from build123d import *

# Parameters (mm, degrees)
SKETCH1_R           = 53.18125
BOSS_EXTRUDE1_DEPTH = 50.8
SKETCH2_R           = 50.8
SKETCH2_R_2         = 47.625
BOSS_EXTRUDE2_DEPTH = 12.7
SKETCH3_R           = 50.00625
CUT_EXTRUDE1_DEPTH  = 53.34
CUT_EXTRUDE1_DRAFT  = -5
SKETCH4_R           = 3.302
CUT_EXTRUDE2_DEPTH  = 93.204372473
SKETCH5_R           = 1.7859375
CUT_EXTRUDE3_DEPTH  = 10.16
CIRPATTERN1_COUNT   = 8


with BuildPart() as part:
    # Sketch1 → Boss-Extrude1 (new body)
    with BuildSketch(Plane(origin=(0, 0, 0), x_dir=(1, 0, 0), z_dir=(0, 1, 0))):
        with Locations(Location((0, 0, 0), (0, 0, 270))):
            Circle(SKETCH1_R)
    extrude(amount=BOSS_EXTRUDE1_DEPTH)

    # Sketch2 → Boss-Extrude2 (add)
    with BuildSketch(Plane.XZ):
        with Locations(Location((0, 0, 0), (0, 0, 270))):
            Circle(SKETCH2_R)
        Circle(SKETCH2_R_2, mode=Mode.SUBTRACT)
        Circle(SKETCH2_R_2)
    extrude(amount=BOSS_EXTRUDE2_DEPTH)


with BuildPart() as cut_extrude1_tool:
    # Sketch3 → Cut-Extrude1 (with draft: the straight prism first)
    with BuildSketch(Plane(origin=(0, 50.8, 0), x_dir=(1, 0, 0), z_dir=(0, 1, 0))):
        Circle(SKETCH3_R)
    extrude(amount=-CUT_EXTRUDE1_DEPTH)
    # Cut-Extrude1: the draft: its side faces are tilted about the plane it starts from
    cut_extrude1_sides = [cut_extrude1_tool.faces().sort_by_distance(p)[0] for p in [
        (-50.00625, 24.13, 0),
    ]]
    draft(cut_extrude1_sides, Plane(origin=(0, 50.8, 0), x_dir=(1, 0, 0), z_dir=(0, 1, 0)), CUT_EXTRUDE1_DRAFT)


with BuildPart() as part_1:
    add(part.part)

    # Cut-Extrude1: cut by cut_extrude1_tool
    add(cut_extrude1_tool.part, mode=Mode.SUBTRACT)

    # Sketch4 → Cut-Extrude2 (cut, through all)
    with BuildSketch(Plane(origin=(0, -2.54, 0), x_dir=(1, 0, 0), z_dir=(0, 1, 0))):
        with Locations(Location((0, 0, 0), (0, 0, 270))):
            Circle(SKETCH4_R)
    extrude(amount=-CUT_EXTRUDE2_DEPTH, mode=Mode.SUBTRACT)

    # Sketch5 → Cut-Extrude3 (cut)
    with BuildSketch(Plane(origin=(50.8, 0, 0), x_dir=(0, 0, -1), z_dir=(1, 0, 0))):
        with Locations((0, -5.35305)):
            Circle(SKETCH5_R)
    cut_extrude3 = extrude(amount=-CUT_EXTRUDE3_DEPTH, mode=Mode.SUBTRACT)

    # CirPattern1: Cut-Extrude3 ×8 about axis
    cirpattern1_axis = Axis((0, 0, 0), (0, 1, 0))
    for i in range(1, CIRPATTERN1_COUNT):
        add(cut_extrude3.rotate(cirpattern1_axis, i * 360 / CIRPATTERN1_COUNT), mode=Mode.SUBTRACT)


solid = part_1.part
For this review, take the finished solid that the model builds, in its own axes (mm). A direction names the side the tool comes from. Give positions to 0.01 mm unless a question says otherwise; leave off trailing zeros. Loops run counter-clockwise (first coordinate to the right, second up) from the corner with the lowest first, then second, coordinate; pieces in that order, holes last. Notation, with made-up numbers: (74, 50.25) -> (114, 50.25) arc R22 ccw to (114, 74.25) -> close; hole circle Ø1 at (78, 88). An arc over 180 degrees is marked (long way). One line per question, with ' | ' between items.
1) We need section A-A (z = 0). Write out the cut boundary in (x, y), plus the area to 3 significant figures.
Resolved:
outline: (-53.18, 0) -> (-50.8, 0) -> (-50.8, -3.57) -> (-40.64, -3.57) -> (-40.64, -7.14) -> (-50.8, -7.14) -> (-50.8, -12.7) -> (-3.3, -12.7) -> (-3.3, -2.54) -> (-45.34, -2.54) -> (-50.01, 50.8) -> (-53.18, 50.8) -> close; (3.3, -12.7) -> (50.8, -12.7) -> (50.8, -7.14) -> (40.64, -7.14) -> (40.64, -3.57) -> (50.8, -3.57) -> (50.8, 0) -> (53.18, 0) -> (53.18, 50.8) -> (50.01, 50.8) -> (45.34, -2.54) -> (3.3, -2.54) -> close | area: 1,470 mm2
2) We need section B-B (x = 0). Write out the cut boundary in (y, z), plus the area to 3 significant figures.
Resolved:
outline: (-12.7, -50.8) -> (-7.14, -50.8) -> (-7.14, -40.64) -> (-3.57, -40.64) -> (-3.57, -50.8) -> (0, -50.8) -> (0, -53.18) -> (50.8, -53.18) -> (50.8, -50.01) -> (-2.54, -45.34) -> (-2.54, -3.3) -> (-12.7, -3.3) -> close; (-12.7, 3.3) -> (-2.54, 3.3) -> (-2.54, 45.34) -> (50.8, 50.01) -> (50.8, 53.18) -> (0, 53.18) -> (0, 50.8) -> (-3.57, 50.8) -> (-3.57, 40.64) -> (-7.14, 40.64) -> (-7.14, 50.8) -> (-12.7, 50.8) -> close | area: 1,470 mm2
3) For faces 4 (the flat face through (0, -5, 40.64)), 5 (the flat face through (40.64, -5, 0)), 6 (the cylindrical face through (-45.79, -6.94, 0.82)), list the 3-axis set-ups (+Z, -Z, +X, -X, +Y, -Y) from which the entire face can be reached by the end or side of a thin tool; tool diameter is ignored.
Resolved:
face 4: +Z | face 5: +X | face 6: -X
4) We need section C-C (y = 11). Write out the cut boundary in (x, z), plus the area to 3 significant figures.
Resolved:
outline: circle Ø106.36 at (0, 0); hole circle Ø93.05 at (0, 0) | area: 2,090 mm2
5) The part is to be moulded in two halves that separate along Z. For faces 1 (the conical face through (-10.229, 18.577, 46.065)), 2 (the flat face through (1, -12.7, -11)), 3 (the flat face through (0, -5, -40.64)), say which applies: +Z half, -Z half, draft (parallel to the pull), parting line (faces both ways), or undercut.
Resolved:
face 1: undercut | face 2: draft | face 3: -Z half
6) To check wall thickness, follow probe 1 along Y at (x, z) = (35.5, 37.5); probe 2 along X at (y, z) = (4, 32); probe 3 along X at (y, z) = (-6, 42). State the ranges of each line that lie inside material, in increasing order.
Resolved:
probe 1: y = 0 to 50.8 | probe 2: x = -42.48 to -32.92, 32.92 to 42.48 | probe 3: x = -28.58 to -1.66, 1.66 to 28.58
7) Insertion check: pin 1 Ø1.8 at (y, z) = (-6, 0.5) entering from -X; pin 2 Ø3 at (y, z) = (20, -12.5) entering from -X; pin 3 Ø6 at (y, z) = (42.5, -36) entering from +X. Each pin has a flat end and moves straight along its axis. Give the tip position at first contact, or say it passes through.
Resolved:
pin 1: stops at x = -40.64 | pin 2: stops at x = -52.03 | pin 3: stops at x = 41.7
8) We need section D-D (y = 46). Write out the cut boundary in (x, z).
Resolved:
outline: circle Ø106.36 at (0, 0); hole circle Ø99.17 at (0, 0)
